from build123d import *

# Parameters (mm, degrees)
BASE_FLANGE1_DEPTH = 185
CUT_EXTRUDE1_REACH = 192.573
SKETCH11_R         = 4
CUT_EXTRUDE2_REACH = 195.916
SKETCH13_R         = 4.5


# Sheet-metal steps are written as plain solids
with BuildPart() as part:
    # Sketch1 → Base-Flange1 (new body)
    with BuildSketch(Plane.XY):
        with BuildLine():
            Line((-20.7, 40.8), (-20.7, 5.6))
            ThreePointArc((-20.7, 5.6), (-19.059797975, 1.640202025), (-15.1, 0))
            Line((-15.1, 0), (15.1, 0))
            ThreePointArc((15.1, 0), (19.059797975, 1.640202025), (20.7, 5.6))
            Line((20.7, 5.6), (20.7, 40.8))
            Line((20.7, 40.8), (17.9, 40.8))
            Line((17.9, 40.8), (17.9, 5.6))
            ThreePointArc((17.9, 5.6), (17.079898987, 3.620101013), (15.1, 2.8))
            Line((15.1, 2.8), (-15.1, 2.8))
            ThreePointArc((-15.1, 2.8), (-17.079898987, 3.620101013), (-17.9, 5.6))
            Line((-17.9, 5.6), (-17.9, 40.8))
            Line((-17.9, 40.8), (-20.7, 40.8))
        make_face()
    extrude(amount=BASE_FLANGE1_DEPTH)

    # Sketch11 → Cut-Extrude1 (cut, up to next)
    with BuildSketch(Plane.XZ, mode=Mode.PRIVATE) as cut_extrude1_sk1:
        with Locations((0, 25)):
            Circle(SKETCH11_R)
    cut_extrude1_tool1 = extrude(cut_extrude1_sk1.sketch, amount=-CUT_EXTRUDE1_REACH, mode=Mode.PRIVATE) & part.part
    add(cut_extrude1_tool1.solids().sort_by_distance((0, 0, 25))[0], mode=Mode.SUBTRACT)

    # Cut-Extrude2: up to this face of the body (flat: up to its plane)
    cut_extrude2_end = Plane(part.part.faces().sort_by_distance((20.7, 23.2, 92.5))[0])
    # Sketch13 → Cut-Extrude2 (cut, up to the picked face)
    with BuildSketch(Plane.ZY.offset(20.7), mode=Mode.PRIVATE) as cut_extrude2_sk1:
        with Locations(Location((50, 27.8, 0), (0, 0, 180))):
            Circle(SKETCH13_R)
    cut_extrude2_tool1 = split(extrude(cut_extrude2_sk1.sketch, amount=-CUT_EXTRUDE2_REACH, mode=Mode.PRIVATE), bisect_by=cut_extrude2_end, keep=Keep.BOTH, mode=Mode.PRIVATE)
    # Sketch13 → Cut-Extrude2 (cut, up to the picked face)
    with BuildSketch(Plane.ZY.offset(20.7), mode=Mode.PRIVATE) as cut_extrude2_sk2:
        with Locations(Location((110, 27.8, 0), (0, 0, 180))):
            Circle(SKETCH13_R)
    cut_extrude2_tool2 = split(extrude(cut_extrude2_sk2.sketch, amount=-CUT_EXTRUDE2_REACH, mode=Mode.PRIVATE), bisect_by=cut_extrude2_end, keep=Keep.BOTH, mode=Mode.PRIVATE)
    # Sketch13 → Cut-Extrude2 (cut, up to the picked face)
    with BuildSketch(Plane.ZY.offset(20.7), mode=Mode.PRIVATE) as cut_extrude2_sk3:
        with Locations(Location((170, 27.8, 0), (0, 0, 180))):
            Circle(SKETCH13_R)
    cut_extrude2_tool3 = split(extrude(cut_extrude2_sk3.sketch, amount=-CUT_EXTRUDE2_REACH, mode=Mode.PRIVATE), bisect_by=cut_extrude2_end, keep=Keep.BOTH, mode=Mode.PRIVATE)
    add(cut_extrude2_tool1.solids().sort_by(Axis((-20.7, 27.8, 50), (1, 0, 0)))[0], mode=Mode.SUBTRACT)
    add(cut_extrude2_tool2.solids().sort_by(Axis((-20.7, 27.8, 110), (1, 0, 0)))[0], mode=Mode.SUBTRACT)
    add(cut_extrude2_tool3.solids().sort_by(Axis((-20.7, 27.8, 170), (1, 0, 0)))[0], mode=Mode.SUBTRACT)


solid = part.part
Design review of the part built by this model. Coordinates are the model's own, in mm. A direction names the side the tool comes from. Coordinates: 2 decimals unless noted, no trailing zeros. Order: outer loops, then holes, each group sorted by start corner. A loop starts at its lowest first (then second) coordinate and runs counter-clockwise, first axis right, second up. Notation, with made-up numbers: (-37.75, 31.5) -> (8.25, 31.5) arc R20 ccw to (8.25, 61.5) -> close; hole circle Ø7 at (77, 26.5). An arc over 180 degrees is marked (long way). One line per item, written item: value.
1) To check wall thickness, follow probe 1 along Z at (x, y) = (19.5, 27.8); probe 2 along X at (y, z) = (24.5, 64); probe 3 along Z at (x, y) = (-18, 27). State the ranges of each line that lie inside material, in increasing order. Write a range as [from, to].
Output values:
probe 1: z = [0, 45.5], [54.5, 105.5], [114.5, 165.5], [174.5, 185]
probe 2: x = [-20.7, -17.9], [17.9, 20.7]
probe 3: z = [0, 45.57], [54.43, 105.57], [114.43, 165.57], [174.43, 185]
2) We need section D-D, the plane z = 170. Give the boundary of the cut face in (x, y).
Output values:
outline: (-20.7, 5.6) arc R5.6 ccw to (-15.1, 0) -> (15.1, 0) arc R5.6 ccw to (20.7, 5.6) -> (20.7, 23.3) -> (17.9, 23.3) -> (17.9, 5.6) arc R2.8 cw to (15.1, 2.8) -> (-15.1, 2.8) arc R2.8 cw to (-17.9, 5.6) -> (-17.9, 23.3) -> (-20.7, 23.3) -> close; (-20.7, 32.3) -> (-17.9, 32.3) -> (-17.9, 40.8) -> (-20.7, 40.8) -> close; (17.9, 32.3) -> (20.7, 32.3) -> (20.7, 40.8) -> (17.9, 40.8) -> close
3) Clearance check with a flat-ended pin moving along its axis: P1, Ø10.5, axis at x = 0, z = 25, coming from the +Y side. State where the tip first meets the part, or that it passes through.
Output values:
P1: stops at y = 2.8
4) We need section C-C, the plane y = 18. Give the boundary of the cut face in (x, z).
Output values:
outline: (-20.7, 0) -> (-17.9, 0) -> (-17.9, 185) -> (-20.7, 185) -> close; (17.9, 0) -> (20.7, 0) -> (20.7, 185) -> (17.9, 185) -> close
5) Machinability: for faces 1 (the face through (0, 2.8, 91)), 2 (the face through (19.02, 1.6, 91.2)), which of the approach directions +Z, -Z, +X, -X, +Y, -Y give a long, thin tool a straight path to every point of the face, cutting with its end or side? Answer none if there is none.
Output values:
face 1: +Z, -Z, +Y
face 2: +Z, -Z, +X, -Y
6) We need section A-A, the plane z = 25. Give the boundary of the cut face in (x, y).
Output values:
outline: (-20.7, 5.6) arc R5.6 ccw to (-15.1, 0) -> (-4, 0) -> (-4, 2.8) -> (-15.1, 2.8) arc R2.8 cw to (-17.9, 5.6) -> (-17.9, 40.8) -> (-20.7, 40.8) -> close; (4, 0) -> (15.1, 0) arc R5.6 ccw to (20.7, 5.6) -> (20.7, 40.8) -> (17.9, 40.8) -> (17.9, 5.6) arc R2.8 cw to (15.1, 2.8) -> (4, 2.8) -> close
7) Draft analysis for pull direction Z (two halves, no side actions). For faces 3 (the face through (-19.32, 27.602, 114.496)), 4 (the face through (0, 0, 91)), 5 (the face through (0, 2, 185)), state which applies: +Z half, -Z half, draft (parallel to the pull), parting line (faces both ways), or undercut.
Output values:
face 3: undercut
face 4: draft
face 5: +Z half
8) We need section B-B, the plane x = 0. Give the boundary of the cut face in (y, z), then the cut area to 3 significant figures.
Output values:
outline: (0, 0) -> (2.8, 0) -> (2.8, 21) -> (0, 21) -> close; (0, 29) -> (2.8, 29) -> (2.8, 185) -> (0, 185) -> close
area: 496 mm2
